```python
from build123d import *

# Parameters (mm, degrees)
SKETCH1_W               = 63.5
SKETCH1_H               = 51.2
BOSS_EXTRUDE1_DEPTH     = 1.65
SKETCH2_W               = 31
SKETCH2_H               = 31
BOSS_EXTRUDE2_DEPTH     = 4.5
SKETCH3_W               = 8.75
SKETCH3_H               = 1.65
CUT_EXTRUDE1_DEPTH      = 1.5
SKETCH4_R               = 4
BOSS_EXTRUDE3_DEPTH     = 1
SKETCH5_R               = 3.1
BOSS_EXTRUDE4_DEPTH     = 6.5
SKETCH6_R               = 1.65
CUT_EXTRUDE2_DEPTH      = 5.5
CUT_EXTRUDE2_DEPTH_BACK = 1.65
BOSS_EXTRUDE5_DEPTH     = 7.3


with BuildPart() as part:
    # Sketch1 → Boss-Extrude1 (new body)
    with BuildSketch(Plane(origin=(0, 0, 0), x_dir=(1, 0, 0), z_dir=(0, 1, 0))):
        with Locations((-1.867647059, -5.657328016)):
            Rectangle(SKETCH1_W, SKETCH1_H)
    extrude(amount=BOSS_EXTRUDE1_DEPTH)

    # Sketch2 → Boss-Extrude2 (add)
    with BuildSketch(Plane(origin=(0, 1.65, 0), x_dir=(1, 0, 0), z_dir=(0, 1, 0))):
        with Locations((-6.617647059, -5.257328016)):
            Rectangle(SKETCH2_W, SKETCH2_H)
    extrude(amount=BOSS_EXTRUDE2_DEPTH)

    # Sketch3 → Cut-Extrude1 (cut)
    with BuildSketch(Plane.ZY.offset(33.617647059)):
        with Locations((-4.817671984, 0.825)):
            Rectangle(SKETCH3_W, SKETCH3_H)
        with Locations((16.132328016, 0.825)):
            Rectangle(SKETCH3_W, SKETCH3_H)
    extrude(amount=-CUT_EXTRUDE1_DEPTH, mode=Mode.SUBTRACT)

    # Sketch4 → Boss-Extrude3 (add)
    with BuildSketch(Plane.ZY.offset(32.117647059)):
        with Locations((-4.817671984, 1.65)):
            Circle(SKETCH4_R)
    boss_extrude3 = extrude(amount=BOSS_EXTRUDE3_DEPTH)

    # Sketch5 → Boss-Extrude4 (add)
    with BuildSketch(Plane.ZY.offset(33.117647059)):
        with Locations((-4.817671984, 1.65)):
            Circle(SKETCH5_R)
    boss_extrude4 = extrude(amount=BOSS_EXTRUDE4_DEPTH)

    # Mirror1: Boss-Extrude3, Boss-Extrude4 across plane
    add(boss_extrude3.mirror(Plane(origin=(0, 0, 5.657328016), x_dir=(1, 0, 0), z_dir=(0, 0, -1))))
    add(boss_extrude4.mirror(Plane(origin=(0, 0, 5.657328016), x_dir=(1, 0, 0), z_dir=(0, 0, -1))))

    # Sketch6 → Cut-Extrude2 (cut, two sides)
    with BuildSketch(Plane(origin=(0, 1.65, 0), x_dir=(1, 0, 0), z_dir=(0, 1, 0))) as cut_extrude2_sk:
        with Locations((-31.067647059, 17.192671984)):
            Circle(SKETCH6_R)
        with Locations((-31.067647059, -28.507328016)):
            Circle(SKETCH6_R)
        with Locations((27.332352941, -28.507328016)):
            Circle(SKETCH6_R)
        with Locations((27.332352941, 17.192671984)):
            Circle(SKETCH6_R)
    extrude(amount=CUT_EXTRUDE2_DEPTH, mode=Mode.SUBTRACT)
    extrude(cut_extrude2_sk.sketch, amount=-CUT_EXTRUDE2_DEPTH_BACK, mode=Mode.SUBTRACT)

    # Sketch7 → Boss-Extrude5 (add)
    with BuildSketch(Plane(origin=(23.982352941, 0, 0), x_dir=(0, 0, -1), z_dir=(1, 0, 0))):
        with BuildLine():
            Line((13.692671984, 1.65), (5.692671984, 1.65))
            ThreePointArc((5.692671984, 1.65), (5.339118593, 1.796446609), (5.192671984, 2.15))
            Line((5.192671984, 2.15), (5.192671984, 4.25))
            ThreePointArc((5.192671984, 4.25), (5.339118593, 4.603553391), (5.692671984, 4.75))
            Line((5.692671984, 4.75), (13.692671984, 4.75))
            ThreePointArc((13.692671984, 4.75), (14.046225375, 4.603553391), (14.192671984, 4.25))
            Line((14.192671984, 4.25), (14.192671984, 2.15))
            ThreePointArc((14.192671984, 2.15), (14.046225375, 1.796446609), (13.692671984, 1.65))
        make_face()
    extrude(amount=BOSS_EXTRUDE5_DEPTH)


solid = part.part
```
Design review of the part built by this model. Coordinates are the model's own, in mm. A direction names the side the tool comes from. Coordinates: 2 decimals unless noted, no trailing zeros. Order: outer loops, then holes, each group sorted by start corner. A loop starts at its lowest first (then second) coordinate and runs counter-clockwise, first axis right, second up. Notation, with made-up numbers: (11.5, 64.25) - (54.5, 64.25) arc R30 cw to (54.5, 100.25) - close; hole circle Ø7 at (7.5, 12). An arc over 180 degrees is marked (long way). One line per question, with ' | ' between items.
Q1. Consider section D-D, the plane z = -2.5. Give the boundary of the cut face in (x, y).
Answer key:
outline: (-39.62, -0.41) - (-33.12, -0.41) - (-33.12, -1.61) - (-32.12, -1.61) - (-32.12, 0) - (29.88, 0) - (29.88, 1.65) - (8.88, 1.65) - (8.88, 6.15) - (-22.12, 6.15) - (-22.12, 1.65) - (-32.12, 1.65) - (-32.12, 4.91) - (-33.12, 4.91) - (-33.12, 3.71) - (-39.62, 3.71) - close
Q2. Clearance check with flat-ended pins moving along their axes: pin 1 Ø5 at (x, y) = (-3, 5) entering from -Z; pin 2 Ø1 at (x, y) = (19.5, -1) entering from +Z; pin 3 Ø1.8 at (y, z) = (1, 27) entering from -X; pin 4 Ø4 at (x, z) = (27.33, -17.19) entering from +Y. State where each tip first meets the part, or that it passes through.
Answer key:
pin 1: stops at z = -10.24 | pin 2: passes through | pin 3: stops at x = -33.62 | pin 4: stops at y = 1.65
Q3. Consider section B-B, the plane y = 3.5. Give the boundary of the cut face in (x, z), then the cut area to 3 significant figures.
Answer key:
outline: (-39.62, -7.31) - (-33.12, -7.31) - (-33.12, -8.36) - (-32.12, -8.36) - (-32.12, -1.27) - (-33.12, -1.27) - (-33.12, -2.33) - (-39.62, -2.33) - close; (-39.62, 13.64) - (-33.12, 13.64) - (-33.12, 12.59) - (-32.12, 12.59) - (-32.12, 19.68) - (-33.12, 19.68) - (-33.12, 18.62) - (-39.62, 18.62) - close; (-22.12, -10.24) - (8.88, -10.24) - (8.88, 20.76) - (-22.12, 20.76) - close; (23.98, -14.19) - (31.28, -14.19) - (31.28, -5.19) - (23.98, -5.19) - close | area: 1,110 mm2
Q4. The part is to be moulded in two halves that separate along X. For faces 6 (the flat face through (-7, 4, 20.757)), 7 (the flat face through (23.982, 3, -10)), 8 (the flat face through (-22.118, 4, 5)), 9 (the flat face through (-33.118, -1, 14)), say which applies: +X half, -X half, draft (parallel to the pull), parting line (faces both ways), or undercut.
Answer key:
face 6: draft | face 7: undercut | face 8: undercut | face 9: -X half
Q5. For faces 1 (the flat face through (28, 3, -14.193)), 2 (the flat face through (28, 4.75, -10)), 3 (the flat face through (-32.118, 3, -5)), 4 (the flat face through (-33, 1, 20.507)), 5 (the flat face through (-33.118, -2, -5)), list the 3-axis set-ups (+Z, -Z, +X, -X, +Y, -Y) from which the entire face can be reached by the end or side of a thin tool; tool diameter is ignored.
Answer key:
face 1: -Z, +X, -X, +Y | face 2: +Z, -Z, +X, +Y | face 3: +Z, -Z, +Y | face 4: -X, +Y, -Y | face 5: -X
Q6. Consider section C-C, the plane z = 22. Give the boundary of the cut face in (x, y).
Answer key:
outline: (-33.62, 0) - (29.88, 0) - (29.88, 1.65) - (-33.62, 1.65) - close
Q7. To check wall thickness, follow line 1 along Z through (x, y) = (-32, 1); line 2 along X through (y, z) = (5.5, -5); line 3 along Z through (x, y) = (0, 3.75). State the ranges of each line that lie inside material, in increasing order.
Answer key:
line 1: z = -19.94 to -18.55, -15.83 to 27.15, 29.87 to 31.26 | line 2: x = -33.12 to -32.12, -22.12 to 8.88 | line 3: z = -10.24 to 20.76
Q8. Consider section A-A, the plane x = 0.5. Give the boundary of the cut face in (y, z).
Answer key:
outline: (0, -19.94) - (1.65, -19.94) - (1.65, -10.24) - (6.15, -10.24) - (6.15, 20.76) - (1.65, 20.76) - (1.65, 31.26) - (0, 31.26) - close
